The figure shows three views and two pictorial views of one solid part (mm, origin at its lowest corner). Answer the questions. Round coordinates to 2 decimals unless told otherwise and drop trailing zeros. Write each loop counter-clockwise with the first axis right and the second up, starting at its lowest first coordinate (ties: lowest second). Pieces come first, ordered by that corner, then holes.
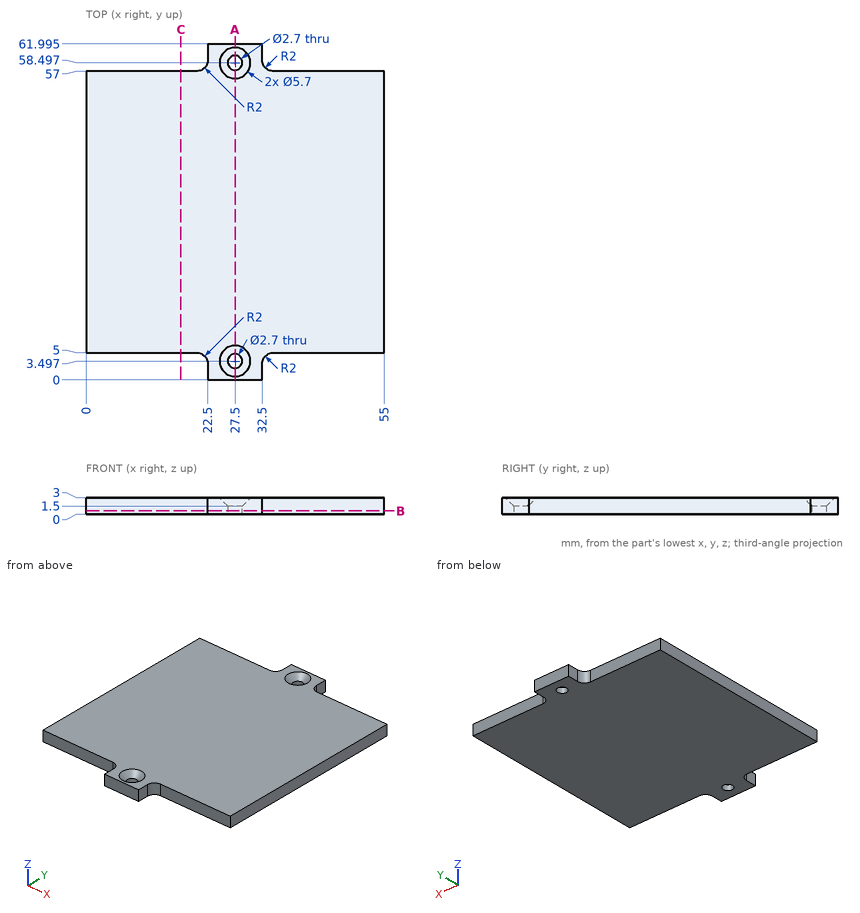
Q1. Section A-A (x = 27.5) is taken. Determine the outline of the cut face in (y, z) (1 decimal).
Verdict:
outline: (0, 0) - (2.1, 0) - (2.1, 1.5) - (0.6, 3) - (0, 3) - close; (4.8, 0) - (57.1, 0) - (57.1, 1.5) - (55.6, 3) - (6.3, 3) - (4.8, 1.5) - close; (59.8, 0) - (62, 0) - (62, 3) - (61.3, 3) - (59.8, 1.5) - close
Q2. Section C-C (x = 17.5) is taken. Determine the outline of the cut face in (y, z).
Verdict:
outline: (5, 0) - (57, 0) - (57, 3) - (5, 3) - close
Q3. Section B-B (z = 0.6) is taken. State how many separate pieces and enclosed holes the cut face has, then the cut area to 3 significant figures.
Verdict:
separate pieces: 1
enclosed holes: 2
area: 2,950 mm2
Q4. Straight lines are drawn through the part: probe 1 along Y at (x, z) = (27.5, 0.7) (1 decimal); probe 2 along X at (y, z) = (58, 2.65); probe 3 along Y at (x, z) = (4, 1.3). For each, find the intervals that lie inside material, in ascending order.
Verdict:
probe 1: y = 0 to 2.1, 4.8 to 57.1, 59.8 to 62
probe 2: x = 22.23 to 25.05, 29.95 to 32.77
probe 3: y = 5 to 57
Q5. Flat-ended cylindrical pins translate along their axes: pin 1 Ø1.5 at (y, z) = (61, 1) entering from -X; pin 2 Ø0.9 at (y, z) = (1.5, 1.5) entering from +X. Find the tip coordinate at first contact, or state that the pin passes through.
Verdict:
pin 1: stops at x = 22.5
pin 2: stops at x = 32.5
